CAD build for the part. Positions are in the model's coordinates, mm. Round coordinates to 2 decimals unless told otherwise and drop trailing zeros. Order: outer loops, then holes, each group sorted by start corner. A loop starts at its lowest first (then second) coordinate and runs counter-clockwise, first axis right, second up.
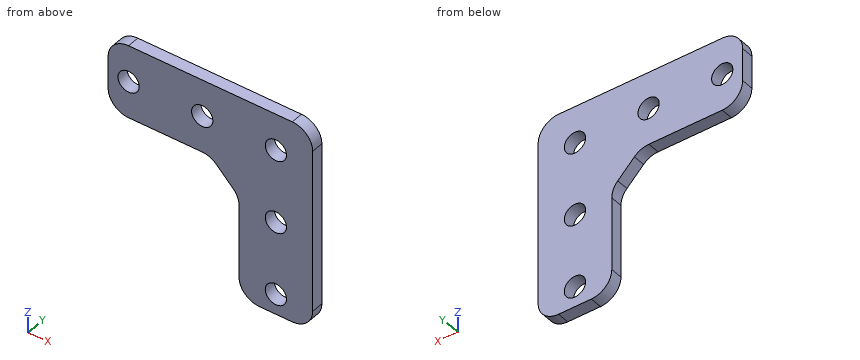
```python
from build123d import *

# Parameters (mm, degrees)
SKETCH1_R          = 2.6
BASE_FLANGE1_DEPTH = 3
FILLET1_R          = 5
FILLET2_R          = 5


# Sheet-metal steps are written as plain solids
with BuildPart() as part:
    # Sketch1 → Base-Flange1 (new body)
    with BuildSketch(Plane(origin=(0, 0, 0), x_dir=(1, 0, 0), z_dir=(0, 1, 0))):
        Polygon((7, 25), (25, 25), (25, -25), (-25, -25), (-25, -7), (0, -7), (7, 0), align=None)
        with Locations(Location((16, -16, 0), (0, 0, 270))):
            Circle(SKETCH1_R, mode=Mode.SUBTRACT)
        with Locations(Location((-2, -16, 0), (0, 0, 270))):
            Circle(SKETCH1_R, mode=Mode.SUBTRACT)
        with Locations(Location((-20, -16, 0), (0, 0, 270))):
            Circle(SKETCH1_R, mode=Mode.SUBTRACT)
        with Locations(Location((16, 2, 0), (0, 0, 270))):
            Circle(SKETCH1_R, mode=Mode.SUBTRACT)
        with Locations(Location((16, 20, 0), (0, 0, 270))):
            Circle(SKETCH1_R, mode=Mode.SUBTRACT)
    extrude(amount=-BASE_FLANGE1_DEPTH)

    # Fillet1
    fillet1_edges = [part.edges().sort_by_distance(p)[0] for p in [
        (0, -1.5, 7),
        (7, -1.5, 0),
    ]]
    fillet(fillet1_edges, radius=FILLET1_R)

    # Fillet2
    fillet2_edges = [part.edges().sort_by_distance(p)[0] for p in [
        (25, -1.5, 25),
        (-25, -1.5, 25),
        (-25, -1.5, 7),
        (7, -1.5, -25),
        (25, -1.5, -25),
    ]]
    fillet(fillet2_edges, radius=FILLET2_R)


solid = part.part
```
1. Cut at A-A, the plane x = 16. Write the cut outline in (y, z), and give its area (3 significant figures).
2. Cut at D-D, the plane z = 0. Write the cut outline in (x, y).
3. Pin check, flat tip, straight feed: P1, Ø1.5, axis at x = -8.5, y = -2, coming from the -Z side. Stop position of the tip, or through.
4. Drill centre lines: line 1 (X direction, y = -0.6, z = 16); line 2 (X direction, y = -1.45, z = -7.5). Where is each one in solid material? Low to high.
5. Cut at C-C, the plane z = 16. Write the cut outline in (x, y).
6. Cut at B-B, the plane y = -2.2. Write the cut outline in (x, z).
Outcome:
1. outline: (-3, -25) - (0, -25) - (0, -22.6) - (-3, -22.6) - close; (-3, -17.4) - (0, -17.4) - (0, -4.6) - (-3, -4.6) - close; (-3, 0.6) - (0, 0.6) - (0, 13.4) - (-3, 13.4) - close; (-3, 18.6) - (0, 18.6) - (0, 25) - (-3, 25) - close
1. area: 103 mm2
2. outline: (6.55, -3) - (14.34, -3) - (14.34, 0) - (6.55, 0) - close; (17.66, -3) - (25, -3) - (25, 0) - (17.66, 0) - close
3. P1: stops at z = 7
4. line 1: x = -25 to -22.6, -17.4 to -4.6, 0.6 to 13.4, 18.6 to 25
4. line 2: x = 7 to 25
5. outline: (-25, -3) - (-22.6, -3) - (-22.6, 0) - (-25, 0) - close; (-17.4, -3) - (-4.6, -3) - (-4.6, 0) - (-17.4, 0) - close; (0.6, -3) - (13.4, -3) - (13.4, 0) - (0.6, 0) - close; (18.6, -3) - (25, -3) - (25, 0) - (18.6, 0) - close
6. outline: (-25, 12) arc R5 ccw to (-20, 7) - (-2.07, 7) arc R5 cw to (1.46, 5.54) - (5.54, 1.46) arc R5 cw to (7, -2.07) - (7, -20) arc R5 ccw to (12, -25) - (20, -25) arc R5 ccw to (25, -20) - (25, 20) arc R5 ccw to (20, 25) - (-20, 25) arc R5 ccw to (-25, 20) - close; hole circle Ø5.2 at (-20, 16); hole circle Ø5.2 at (-2, 16); hole circle Ø5.2 at (16, -20); hole circle Ø5.2 at (16, -2); hole circle Ø5.2 at (16, 16)
